Here's the drawing with two shaded views (mm, measured from the low corner). I have some questions. Give positions to 0.01 mm unless a question says otherwise; leave off trailing zeros. Loops run counter-clockwise (first coordinate to the right, second up) from the corner with the lowest first, then second, coordinate; pieces in that order, holes last. Notation, with made-up numbers: M 49,13.5 L 102,13.5 A12 ccw 102,22.5 Z; hole C 66.25,6 d3. An arc over 180 degrees is marked long. Use CSV: the item, a comma, the result in double quotes.
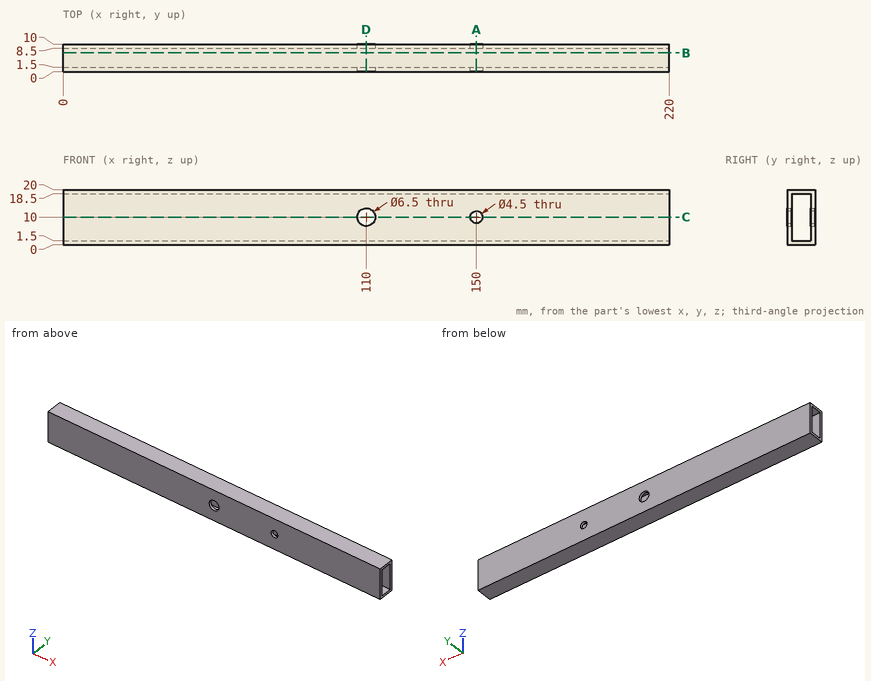
1. I want a section at C-C, the plane z = 10. List the corners of the cut face in (x, y) for me, then the cut area to 3 significant figures.
Outcome:
outline,"M 0,0 L 106.75,0 L 106.75,1.5 L 0,1.5 Z; M 0,8.5 L 106.75,8.5 L 106.75,10 L 0,10 Z; M 113.25,0 L 147.75,0 L 147.75,1.5 L 113.25,1.5 Z; M 113.25,8.5 L 147.75,8.5 L 147.75,10 L 113.25,10 Z; M 152.25,0 L 220,0 L 220,1.5 L 152.25,1.5 Z; M 152.25,8.5 L 220,8.5 L 220,10 L 152.25,10 Z"
area,"627 mm2"
2. Please list where these lines run through material, in increasing order: line 1 (X direction, y = 9.25, z = 10); line 2 (Y direction, x = 153.5, z = 7); line 3 (Z direction, x = 150, y = 0.6).
Outcome:
line 1,"0 to 106.75, 113.25 to 147.75, 152.25 to 220"
line 2,"0 to 1.5, 8.5 to 10"
line 3,"0 to 7.75, 12.25 to 20"
3. I want a section at A-A, the plane x = 150. List the corners of the cut face in (y, z) for me, then the cut area to 3 significant figures.
Outcome:
outline,"M 0,0 L 10,0 L 10,7.75 L 8.5,7.75 L 8.5,1.5 L 1.5,1.5 L 1.5,7.75 L 0,7.75 Z; M 0,12.25 L 1.5,12.25 L 1.5,18.5 L 8.5,18.5 L 8.5,12.25 L 10,12.25 L 10,20 L 0,20 Z"
area,"67.5 mm2"
4. I want a section at D-D, the plane x = 110. List the corners of the cut face in (y, z) for me, then the cut area to 3 significant figures.
Outcome:
outline,"M 0,0 L 10,0 L 10,6.75 L 8.5,6.75 L 8.5,1.5 L 1.5,1.5 L 1.5,6.75 L 0,6.75 Z; M 0,13.25 L 1.5,13.25 L 1.5,18.5 L 8.5,18.5 L 8.5,13.25 L 10,13.25 L 10,20 L 0,20 Z"
area,"61.5 mm2"
5. I want a section at B-B, the plane y = 6.75. List the corners of the cut face in (x, z) for me.
Outcome:
outline,"M 0,0 L 220,0 L 220,1.5 L 0,1.5 Z; M 0,18.5 L 220,18.5 L 220,20 L 0,20 Z"
